Verification items for the finished model (mm, model axes). Face numbers are marked on the shaded views. A direction names the side the tool comes from. Round coordinates to 2 decimals unless told otherwise and drop trailing zeros. Write each loop counter-clockwise with the first axis right and the second up, starting at its lowest first coordinate (ties: lowest second). Pieces come first, ordered by that corner, then holes. Notation, with made-up numbers: (29, -10) -> (51, -10) arc R22 cw to (51, 11) -> close; hole circle Ø8 at (-23, -3). An arc over 180 degrees is marked (long way). Use CSV: the item, a comma, the result in double quotes.
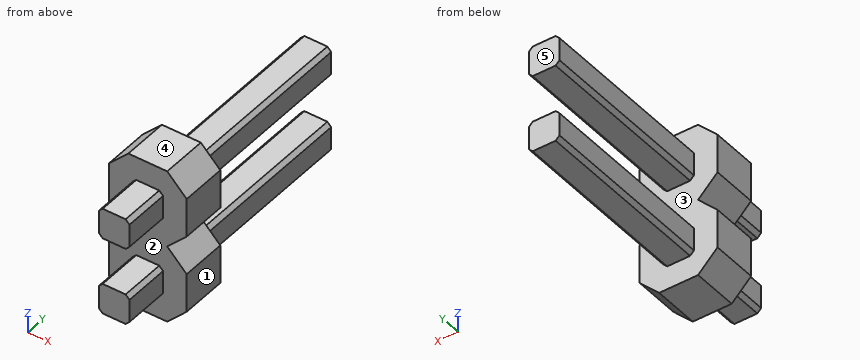
```python
from build123d import *

# Parameters (mm, degrees)
BOSS_EXTRUDE1_DEPTH      = 1.5
BOSS_EXTRUDE2_DEPTH      = 6
BOSS_EXTRUDE2_DEPTH_BACK = 3
CUT_EXTRUDE1_DEPTH       = 13.69206445
CUT_EXTRUDE1_DEPTH_BACK  = 13.69206445
CUT_EXTRUDE2_DEPTH       = 6
CUT_EXTRUDE2_DEPTH_BACK  = 6


with BuildPart() as part:
    # Sketch1 → Boss-Extrude1 (new body)
    with BuildSketch(Plane(origin=(0, 0, 0), x_dir=(1, 0, 0), z_dir=(0, 1, 0))):
        Polygon((-0.635, 10.16), (0.635, 10.16), (1.27, 9.525), (1.27, 8.255), (0.635, 7.62), (1.27, 6.985), (1.27, 5.715), (0.635, 5.08), (1.27, 4.445), (1.27, 3.175), (0.635, 2.54), (1.27, 1.905), (1.27, 0.635), (0.635, 0), (1.27, -0.635), (1.27, -1.905), (0.635, -2.54), (1.27, -3.175), (1.27, -4.445), (0.635, -5.08), (-0.635, -5.08), (-1.27, -4.445), (-1.27, -3.175), (-0.635, -2.54), (-1.27, -1.905), (-1.27, -0.635), (-0.635, 0), (-1.27, 0.635), (-1.27, 1.905), (-0.635, 2.54), (-1.27, 3.175), (-1.27, 4.445), (-0.635, 5.08), (-1.27, 5.715), (-1.27, 6.985), (-0.635, 7.62), (-1.27, 8.255), (-1.27, 9.525), align=None)
    extrude(amount=BOSS_EXTRUDE1_DEPTH)

    # Sketch3 → Boss-Extrude2 (add, two sides: drawn at the far end of the back side and taken through both)
    with BuildSketch(Plane(origin=(0, 1.5, 0), x_dir=(1, 0, 0), z_dir=(0, 1, 0)).offset(-BOSS_EXTRUDE2_DEPTH_BACK)):
        Polygon((0.375, 9.39), (0.5, 9.265), (0.5, 8.515), (0.375, 8.39), (-0.375, 8.39), (-0.5, 8.515), (-0.5, 9.265), (-0.375, 9.39), align=None)
        Polygon((0.375, 6.85), (0.5, 6.725), (0.5, 5.975), (0.375, 5.85), (-0.375, 5.85), (-0.5, 5.975), (-0.5, 6.725), (-0.375, 6.85), align=None)
        Polygon((0.375, 4.31), (0.5, 4.185), (0.5, 3.435), (0.375, 3.31), (-0.375, 3.31), (-0.5, 3.435), (-0.5, 4.185), (-0.375, 4.31), align=None)
        Polygon((0.375, 1.77), (0.5, 1.645), (0.5, 0.895), (0.375, 0.77), (-0.375, 0.77), (-0.5, 0.895), (-0.5, 1.645), (-0.375, 1.77), align=None)
        Polygon((0.375, -0.77), (0.5, -0.895), (0.5, -1.645), (0.375, -1.77), (-0.375, -1.77), (-0.5, -1.645), (-0.5, -0.895), (-0.375, -0.77), align=None)
        Polygon((0.375, -3.31), (0.5, -3.435), (0.5, -4.185), (0.375, -4.31), (-0.375, -4.31), (-0.5, -4.185), (-0.5, -3.435), (-0.375, -3.31), align=None)
    extrude(amount=BOSS_EXTRUDE2_DEPTH + BOSS_EXTRUDE2_DEPTH_BACK)

    # Sketch4 → Cut-Extrude1 (cut, two sides: drawn at the far end of the back side and taken through both)
    with BuildSketch(Plane(origin=(0, 0, 0), x_dir=(1, 0, 0), z_dir=(0, 1, 0)).offset(-CUT_EXTRUDE1_DEPTH_BACK)):
        Polygon((0.635, 2.54), (-0.635, 2.54), (-3.551273802, 2.145414022), (-3.551273802, -5.54901255), (3.518391637, -6.305302341), (3.518391637, 1.323359901), align=None)
    extrude(amount=CUT_EXTRUDE1_DEPTH + CUT_EXTRUDE1_DEPTH_BACK, mode=Mode.SUBTRACT)

    # Sketch5 → Cut-Extrude2 (cut, two sides: drawn at the far end of the back side and taken through both)
    with BuildSketch(Plane(origin=(0, 1.5, 0), x_dir=(1, 0, 0), z_dir=(0, 1, 0)).offset(-CUT_EXTRUDE2_DEPTH_BACK)):
        Polygon((-0.635, 7.62), (0.635, 7.62), (3.304657566, 8.536663962), (1.969828783, 11.132382054), (-2.565180809, 11.132382054), (-2.565180809, 10.824604991), (-2.565180809, 7.895726944), align=None)
    extrude(amount=CUT_EXTRUDE2_DEPTH + CUT_EXTRUDE2_DEPTH_BACK, mode=Mode.SUBTRACT)


solid = part.part
```
Q1. Mould release check, pull along Z, two halves, no side actions. Record for the marked faces 3, 4 and 5: released by +Z, released by -Z, zero draft, split by the parting line, or undercut.
Filled in:
face 3,"undercut"
face 4,"released by +Z"
face 5,"zero draft"
Q2. Material ranges on L1, parallel to Z at x = 0.3, y = 3; L2, parallel to Y at x = 1, z = -4.2; L3, parallel to X at y = 5.5, z = -3.9, recorded low to high.
Filled in:
L1,"-6.85 to -5.85, -4.31 to -3.31"
L2,"0 to 1.5"
L3,"-0.5 to 0.5"
Q3. Section check B-B (x = 0.75). Record the cut outline in (y, z) (3 decimals), plus the area to 3 significant figures.
Filled in:
outline,"(0, -7.505) -> (1.5, -7.505) -> (1.5, -5.195) -> (0, -5.195) -> close; (0, -4.965) -> (1.5, -4.965) -> (1.5, -2.655) -> (0, -2.655) -> close"
area,"6.93 mm²"
Q4. Section check A-A (y = 5.5). Record the cut outline in (x, z) (3 decimals).
Filled in:
outline,"(-0.5, -6.725) -> (-0.375, -6.85) -> (0.375, -6.85) -> (0.5, -6.725) -> (0.5, -5.975) -> (0.375, -5.85) -> (-0.375, -5.85) -> (-0.5, -5.975) -> close; (-0.5, -4.185) -> (-0.375, -4.31) -> (0.375, -4.31) -> (0.5, -4.185) -> (0.5, -3.435) -> (0.375, -3.31) -> (-0.375, -3.31) -> (-0.5, -3.435) -> close"
Q5. Section check C-C (z = -3.95). Record the cut outline in (x, y), plus the area to 3 significant figures.
Filled in:
outline,"(-1.27, 0) -> (-0.5, 0) -> (-0.5, -1.5) -> (0.5, -1.5) -> (0.5, 0) -> (1.27, 0) -> (1.27, 1.5) -> (0.5, 1.5) -> (0.5, 7.5) -> (-0.5, 7.5) -> (-0.5, 1.5) -> (-1.27, 1.5) -> close"
area,"11.3 mm²"
Q6. Access from +Z, -Z, +X, -X, +Y, -Y to the whole of each face (thin tool, end or side, straight path). Record for the marked faces 1 and 2.
Filled in:
face 1,"+Z, -Z, +X, +Y, -Y"
face 2,"-Y"
Q7. Go/stop test with flat-tipped pins: P1, Ø0.6, axis at y = -0.5, z = -6.5, coming from the +X side; P2, Ø0.6, axis at y = -0.5, z = -6, coming from the -X side; P3, Ø1.5, axis at x = 0.5, z = -5, coming from the +Y side; P4, Ø1.5, axis at x = -1, y = 6.5, coming from the +Z side. Record where each tip stops, or that it passes through.
Filled in:
P1,"x = 0.5"
P2,"x = -0.5"
P3,"y = 7.5"
P4,"z = -3.31"
Q8. Section check D-D (y = 0.75). Record the cut outline in (x, z) (3 decimals).
Filled in:
outline,"(-1.27, -6.985) -> (-0.635, -7.62) -> (0.635, -7.62) -> (1.27, -6.985) -> (1.27, -5.715) -> (0.635, -5.08) -> (1.27, -4.445) -> (1.27, -3.175) -> (0.635, -2.54) -> (-0.635, -2.54) -> (-1.27, -3.175) -> (-1.27, -4.445) -> (-0.635, -5.08) -> (-1.27, -5.715) -> close"
